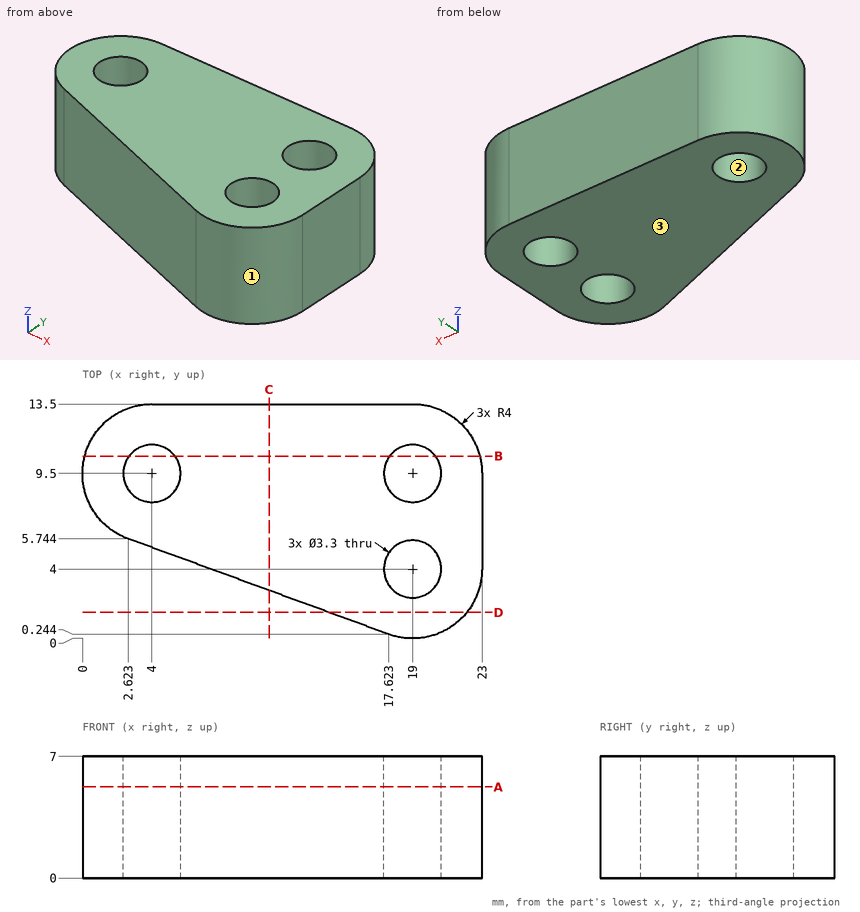
Print and shaded views of the part. All mm, measured from the part's lowest x, y and z. Give positions to 0.01 mm unless a question says otherwise; leave off trailing zeros. Loops run counter-clockwise (first coordinate to the right, second up) from the corner with the lowest first, then second, coordinate; pieces in that order, holes last. Notation, with made-up numbers: (58.5, 1) - (86.5, 1) arc R15 cw to (86.5, 28) - close; hole circle Ø2 at (63.25, 65.5). An arc over 180 degrees is marked (long way). Use a Markdown table: item, result.
(1) Drop flat-ended pins along their axis: pin 1 Ø3 at (x, z) = (5.5, 2) entering from -Y; pin 2 Ø1 at (x, z) = (9, 5.5) entering from -Y. Give the stop position or say it passes through.
Taken from the geometry:
| item | result |
|---|---|
| pin 1 | y = 4.14 |
| pin 2 | y = 3.22 |
(2) Band-saw the part on C-C (x = 10.75). Give the cut face in (y, z) (1 decimal).
Taken from the geometry:
| item | result |
|---|---|
| outline | (2.8, 0) - (13.5, 0) - (13.5, 7) - (2.8, 7) - close |
(3) Pull direction X, two halves, no side cores. Call the marked faces 1, 2 and 3: +X half, -X half, draft (parallel to the pull), parting line (faces both ways), or undercut.
Taken from the geometry:
| item | result |
|---|---|
| face 1 | parting line |
| face 2 | undercut |
| face 3 | draft |
(4) Band-saw the part on A-A (z = 5.25). Give the number of separate pieces and of enclosed holes in the cut face, and give its area (3 significant figures).
Taken from the geometry:
| item | result |
|---|---|
| separate pieces | 1 |
| enclosed holes | 3 |
| area | 212 mm2 |
(5) Band-saw the part on D-D (y = 1.5). Give the cut face in (x, z).
Taken from the geometry:
| item | result |
|---|---|
| outline | (14.2, 0) - (22.12, 0) - (22.12, 7) - (14.2, 7) - close |
(6) Band-saw the part on B-B (y = 10.5). Give the cut face in (x, z).
Taken from the geometry:
| item | result |
|---|---|
| outline | (0.13, 0) - (2.69, 0) - (2.69, 7) - (0.13, 7) - close; (5.31, 0) - (17.69, 0) - (17.69, 7) - (5.31, 7) - close; (20.31, 0) - (22.87, 0) - (22.87, 7) - (20.31, 7) - close |
(7) Wall check: line 1 along Y through (x, z) = (19, 3); line 2 along X through (y, z) = (8, 4.75) (1 decimal); line 3 along Y through (x, z) = (17.5, 2) (1 decimal). Give the ranges that are in metal, low to high.
Taken from the geometry:
| item | result |
|---|---|
| line 1 | 0 to 2.35, 5.65 to 7.85, 11.15 to 13.5 |
| line 2 | 0.3 to 3.3, 4.7 to 18.3, 19.7 to 23 |
| line 3 | 0.3 to 3.3, 4.7 to 8.8, 10.2 to 13.5 |
